Autodesk Inventor part; units mm, degrees
ref_plane "YZ Plane" through (0, 0, 0) normal (1, 0, 0) x (0, 1, 0)
ref_plane "XZ Plane" through (0, 0, 0) normal (0, 1, 0) x (-1, 0, 0)
ref_plane "XY Plane" through (0, 0, 0) normal (0, 0, 1) x (1, 0, 0)
sketch "Sketch1" plane through (0, 0, 0) normal (0, 1, 0) x (-1, 0, 0)
  circle A0 centre (0, 0) radius 97.5
  circle A1 centre (0, 0) radius 111.25
  dimension "d0" = 195
  dimension "d1" = 222.5
extrude "Extrusion1" add sketch "Sketch1" along normal blind 10
sketch "Sketch2" plane through (0, 10, 0) normal (0, 1, 0) x (1, 0, 0)
  line L0 (0, 0) -> (0, 104.375)
  dimension "d4" = 104.375
hole "Hole1" at (0, 10, -104.375) direction (0, -1, 0) diameter 2.5 end through all countersink diameter 5 countersink angle 90
pattern_circular "Circular Pattern1" count 4 over 360 about axis through (0, -10, 0) along (0, 1, 0) of "Hole1"
sketch "Sketch3" plane through (0, 10, 0) normal (0, 1, 0) x (1, 0, 0)
  circle A0 centre (-104.375, 0) radius 1.25
  line L0 (-104.375, 0) -> (0, 0)
  circle A1 centre (0, 104.375) radius 1.25
  line L1 (0, 0) -> (0, 104.375)
  line L2 (0, 104.375) -> (-104.375, 0)
properties part number "InnerBearingTable"
Source: CAD feature listing. Evaluate the final solid. Frame: model axes, mm. Coordinates: 2 decimals unless noted, no trailing zeros. Loops run counter-clockwise (first coordinate to the right, second up) from the corner with the lowest first, then second, coordinate; pieces in that order, holes last. Notation, with made-up numbers: (-28, 78.5) - (-7, 78.5) arc R25 ccw to (-7, 103.5) - close; hole circle Ø7 at (9.5, 34). An arc over 180 degrees is marked (long way). Return JSON: item names as keys, results as strings.
Q1. Section B-B, the plane z = 74. Return loops of the section in (x, y).
Results:
{"outline": "(-83.07, 0) - (-63.48, 0) - (-63.48, 10) - (-83.07, 10) - close; (63.48, 0) - (83.07, 0) - (83.07, 10) - (63.48, 10) - close"}
Q2. Material intervals for line 1 along X through (y, z) = (5.5, 54.5); line 2 along X through (y, z) = (6.5, -17); line 3 along Z through (x, y) = (28, 8.75), sorted ascending.
Results:
{"line 1": "-96.99 to -80.85, 80.85 to 96.99", "line 2": "-109.94 to -96.01, 96.01 to 109.94", "line 3": "-107.67 to -93.39, 93.39 to 107.67"}
Q3. Contact query for flat-ended pins moving along their axis: P1, Ø1.5, axis at x = 0, z = 104.375, coming from the +Y side; P2, Ø3, axis at y = 2, z = 64.5, coming from the -X side; P3, Ø4, axis at y = 4, z = -71, coming from the -X side; P4, Ø3, axis at x = -29.5, y = 2.5, coming from the -Z side. Output: stop coordinate, or through.
Results:
{"P1": "through", "P2": "x = -91.69", "P3": "x = -87.27", "P4": "z = -107.67"}
Q4. Section C-C, the plane y = 6. Return loops of the section in (x, z) (3 decimals), plus the area to 3 significant figures.
Results:
{"outline": "circle Ø222.5 at (0, 0); hole circle Ø2.5 at (-104.375, 0); hole circle Ø195 at (0, 0); hole circle Ø2.5 at (0, -104.375); hole circle Ø2.5 at (0, 104.375); hole circle Ø2.5 at (104.375, 0)", "area": "9,000 mm2"}
Q5. Mould query, pull axis X, two halves, no side actions, for faces 1 (the cylindrical face through (14.5, 4.9, -110.3)), 2 (the flat face through (1, 10, -98)), 3 (the cylindrical face through (77.37, 4.93, 59.33)). Classes: released by +X, released by -X, zero draft, split by the parting line, or undercut.
Results:
{"face 1": "split by the parting line", "face 2": "zero draft", "face 3": "undercut"}
Q6. Section A-A, the plane x = 71.5. Return loops of the section in (y, z).
Results:
{"outline": "(0, -85.23) - (10, -85.23) - (10, -66.29) - (0, -66.29) - close; (0, 66.29) - (10, 66.29) - (10, 85.23) - (0, 85.23) - close"}
